```python
from build123d import *

# Parameters (mm, degrees)
RESSALTO_EXTRUS_O1_DEPTH = 3


with BuildPart() as part:
    # Esboço1 → Ressalto-extrusão1 (new body)
    with BuildSketch(Plane.XY):
        Polygon((-80.141377403, 21.254023913), (-83.141377403, 21.254023913), (-83.141377403, -8.745976087), (-80.141377403, -8.745976087), (-80.141377403, -38.745976087), (-83.141377403, -38.745976087), (-83.141377403, -68.745976087), (-80.141377403, -68.745976087), (-80.141377403, -98.745976087), (-83.141377403, -98.745976087), (-83.141377403, -128.745976087), (-80.141377403, -128.745976087), (-80.141377403, -131.677493187), (-50.141377403, -131.677493187), (-50.141377403, -128.677493187), (-20.141377403, -128.677493187), (-20.141377403, -131.677493187), (9.858622597, -131.677493187), (9.858622597, -128.677493187), (40.700385396, -128.677493187), (40.700385396, -131.677493187), (70.700385396, -131.677493187), (70.700385396, -128.745976087), (73.700385396, -128.745976087), (73.700385396, -98.745976087), (70.700385396, -98.745976087), (70.700385396, -68.745976087), (73.700385396, -68.745976087), (73.700385396, -38.745976087), (70.700385396, -38.745976087), (70.700385396, -8.745976087), (72.858622597, -8.745976087), (72.858622597, 21.254023913), (69.858622597, 21.254023913), (69.858622597, 24.322506813), (39.858622597, 24.322506813), (39.858622597, 21.322506813), (9.858622597, 21.322506813), (9.858622597, 24.322506813), (-20.141377403, 24.322506813), (-20.141377403, 21.322506813), (-50.141377403, 21.322506813), (-50.141377403, 24.322506813), (-80.141377403, 24.322506813), align=None)
        with BuildLine():
            Line((35.066575056, -21.699226817), (25.066575056, -21.699226817))
            ThreePointArc((25.066575056, -21.699226817), (20.066575056, -16.699226817), (25.066575056, -11.699226817))
            Line((25.066575056, -11.699226817), (35.066575056, -11.699226817))
            ThreePointArc((35.066575056, -11.699226817), (40.066575056, -16.699226817), (35.066575056, -21.699226817))
        make_face(mode=Mode.SUBTRACT)
        with BuildLine():
            Line((-0.141377403, -21.699226817), (-10.141377403, -21.699226817))
            ThreePointArc((-10.141377403, -21.699226817), (-15.141377403, -16.699226817), (-10.141377403, -11.699226817))
            Line((-10.141377403, -11.699226817), (-0.141377403, -11.699226817))
            ThreePointArc((-0.141377403, -11.699226817), (4.858622597, -16.699226817), (-0.141377403, -21.699226817))
        make_face(mode=Mode.SUBTRACT)
        with BuildLine():
            Line((-35.141377403, -21.699226817), (-45.141377403, -21.699226817))
            ThreePointArc((-45.141377403, -21.699226817), (-50.141377403, -16.699226817), (-45.141377403, -11.699226817))
            Line((-45.141377403, -11.699226817), (-35.141377403, -11.699226817))
            ThreePointArc((-35.141377403, -11.699226817), (-30.141377403, -16.699226817), (-35.141377403, -21.699226817))
        make_face(mode=Mode.SUBTRACT)
        with BuildLine():
            Line((35.066575056, -58.745976087), (25.066575056, -58.745976087))
            ThreePointArc((25.066575056, -58.745976087), (20.066575056, -53.745976087), (25.066575056, -48.745976087))
            Line((25.066575056, -48.745976087), (35.066575056, -48.745976087))
            ThreePointArc((35.066575056, -48.745976087), (40.066575056, -53.745976087), (35.066575056, -58.745976087))
        make_face(mode=Mode.SUBTRACT)
        with BuildLine():
            Line((-0.141377403, -58.745976087), (-10.141377403, -58.745976087))
            ThreePointArc((-10.141377403, -58.745976087), (-15.141377403, -53.745976087), (-10.141377403, -48.745976087))
            Line((-10.141377403, -48.745976087), (-0.141377403, -48.745976087))
            ThreePointArc((-0.141377403, -48.745976087), (4.858622597, -53.745976087), (-0.141377403, -58.745976087))
        make_face(mode=Mode.SUBTRACT)
        with BuildLine():
            Line((-35.141377403, -58.745976087), (-45.141377403, -58.745976087))
            ThreePointArc((-45.141377403, -58.745976087), (-50.141377403, -53.745976087), (-45.141377403, -48.745976087))
            Line((-45.141377403, -48.745976087), (-35.141377403, -48.745976087))
            ThreePointArc((-35.141377403, -48.745976087), (-30.141377403, -53.745976087), (-35.141377403, -58.745976087))
        make_face(mode=Mode.SUBTRACT)
        with BuildLine():
            Line((35.066575056, -93.745976087), (25.066575056, -93.745976087))
            ThreePointArc((25.066575056, -93.745976087), (20.066575056, -88.745976087), (25.066575056, -83.745976087))
            Line((25.066575056, -83.745976087), (35.066575056, -83.745976087))
            ThreePointArc((35.066575056, -83.745976087), (40.066575056, -88.745976087), (35.066575056, -93.745976087))
        make_face(mode=Mode.SUBTRACT)
        with BuildLine():
            Line((-0.141377403, -93.745976087), (-10.141377403, -93.745976087))
            ThreePointArc((-10.141377403, -93.745976087), (-15.141377403, -88.745976087), (-10.141377403, -83.745976087))
            Line((-10.141377403, -83.745976087), (-0.141377403, -83.745976087))
            ThreePointArc((-0.141377403, -83.745976087), (4.858622597, -88.745976087), (-0.141377403, -93.745976087))
        make_face(mode=Mode.SUBTRACT)
        with BuildLine():
            Line((-35.141377403, -93.745976087), (-45.141377403, -93.745976087))
            ThreePointArc((-45.141377403, -93.745976087), (-50.141377403, -88.745976087), (-45.141377403, -83.745976087))
            Line((-45.141377403, -83.745976087), (-35.141377403, -83.745976087))
            ThreePointArc((-35.141377403, -83.745976087), (-30.141377403, -88.745976087), (-35.141377403, -93.745976087))
        make_face(mode=Mode.SUBTRACT)
    extrude(amount=RESSALTO_EXTRUS_O1_DEPTH)


solid = part.part
```
Design review of the part built by this model. Coordinates are the model's own, in mm. Coordinates: 2 decimals unless noted, no trailing zeros. Order: outer loops, then holes, each group sorted by start corner. A loop starts at its lowest first (then second) coordinate and runs counter-clockwise, first axis right, second up. Notation, with made-up numbers: (-34.75, 48) - (13.25, 48) arc R16 cw to (13.25, 74) - close; hole circle Ø4 at (53, 19). An arc over 180 degrees is marked (long way). One line per question, with ' | ' between items.
Q1. The part is to be moulded in two halves that separate along X. For faces 1 (the flat face through (-6, -70, 0)), 2 (the cylindrical face through (40.065, -88.636, 1.479)), say which applies: +X half, -X half, draft (parallel to the pull), parting line (faces both ways), or undercut.
Answer key:
face 1: draft | face 2: undercut
Q2. To check wall thickness, follow line 1 along Y through (x, z) = (-2.5, 1.85); line 2 along Y through (x, z) = (27, 2.2); line 3 along X through (y, z) = (-25.5, 0.85). State the ranges of each line that lie inside material, in increasing order.
Answer key:
line 1: y = -131.68 to -93.75, -83.75 to -58.75, -48.75 to -21.7, -11.7 to 24.32 | line 2: y = -128.68 to -93.75, -83.75 to -58.75, -48.75 to -21.7, -11.7 to 21.32 | line 3: x = -80.14 to 70.7
Q3. Consider section B-B, the plane y = -56. Give the boundary of the cut face in (x, z).
Answer key:
outline: (-83.14, 0) - (-49.6, 0) - (-49.6, 3) - (-83.14, 3) - close; (-30.68, 0) - (-14.6, 0) - (-14.6, 3) - (-30.68, 3) - close; (4.32, 0) - (20.6, 0) - (20.6, 3) - (4.32, 3) - close; (39.53, 0) - (73.7, 0) - (73.7, 3) - (39.53, 3) - close
Q4. Consider section C-C, the plane z = 0.85. Give the number of separate pieces and of enclosed holes in the cut face, then the cut area to 3 significant figures.
Answer key:
separate pieces: 1 | enclosed holes: 9 | area: 22,100 mm2
Q5. Clearance check with flat-ended pins moving along their axes: pin 1 Ø0.9 at (x, z) = (-39, 1.5) entering from +Y; pin 2 Ø1.5 at (y, z) = (-130, 1) entering from +X. State where each tip first meets the part, or that it passes through.
Answer key:
pin 1: stops at y = 21.32 | pin 2: stops at x = 70.7
Q6. Consider section A-A, the plane x = -41. Give the boundary of the cut face in (y, z), then the cut area to 3 significant figures.
Answer key:
outline: (-128.68, 0) - (-93.75, 0) - (-93.75, 3) - (-128.68, 3) - close; (-83.75, 0) - (-58.75, 0) - (-58.75, 3) - (-83.75, 3) - close; (-48.75, 0) - (-21.7, 0) - (-21.7, 3) - (-48.75, 3) - close; (-11.7, 0) - (21.32, 0) - (21.32, 3) - (-11.7, 3) - close | area: 360 mm2
